Geometry check sheet. Reference: drawing and pictorial views, mm from the part's lowest x, y, z. Give positions to 0.01 mm unless a question says otherwise; leave off trailing zeros. Order: outer loops, then holes, each group sorted by start corner. A loop starts at its lowest first (then second) coordinate and runs counter-clockwise, first axis right, second up. Notation, with made-up numbers: M 63.5,76 L 83.5,76 A33 cw 83.5,111 Z; hole C -25.5,13 d9. An arc over 180 degrees is marked long. Answer as CSV lines item,"result".
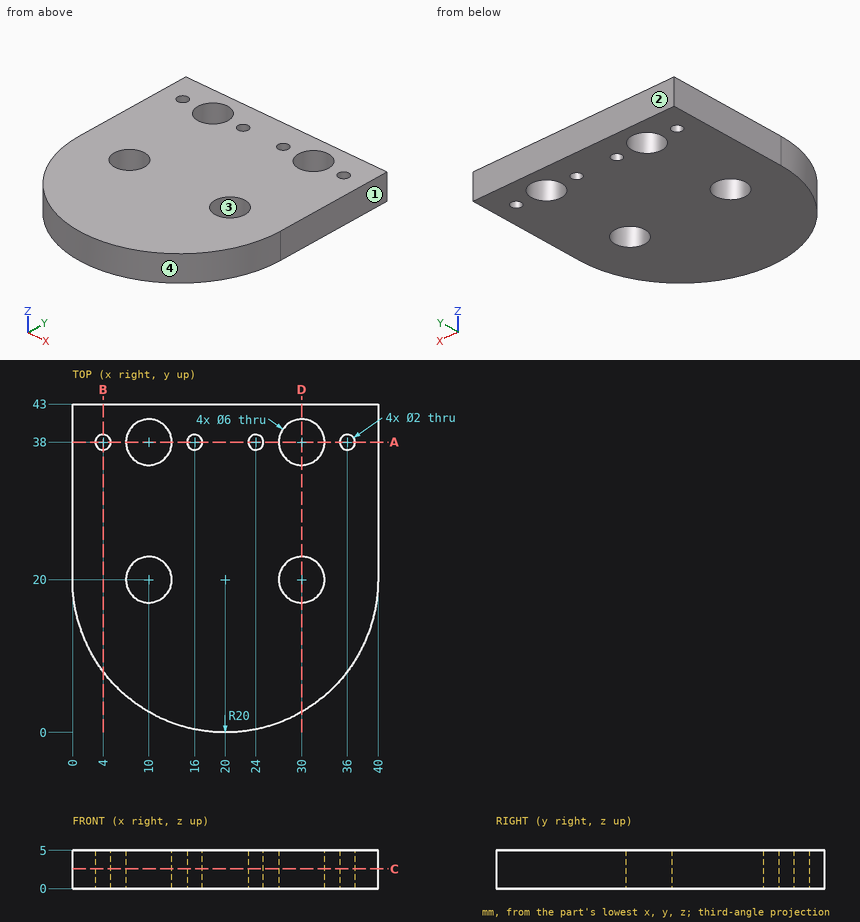
(1) Section check C-C on z = 2.6. State how many separate pieces and enclosed holes the cut face has, then the cut area to 3 significant figures.
The answers:
separate pieces,"1"
enclosed holes,"8"
area,"1,420 mm2"
(2) Section check A-A on y = 38. Enter the section's corners in (x, z).
The answers:
outline,"M 0,0 L 3,0 L 3,5 L 0,5 Z; M 5,0 L 7,0 L 7,5 L 5,5 Z; M 13,0 L 15,0 L 15,5 L 13,5 Z; M 17,0 L 23,0 L 23,5 L 17,5 Z; M 25,0 L 27,0 L 27,5 L 25,5 Z; M 33,0 L 35,0 L 35,5 L 33,5 Z; M 37,0 L 40,0 L 40,5 L 37,5 Z"
(3) Draft check along X on the marked faces 1, 2, 3 and 4. Enter one of: +X half, -X half, draft (parallel to the pull), parting line (faces both ways), or undercut.
The answers:
face 1,"+X half"
face 2,"draft"
face 3,"undercut"
face 4,"parting line"
(4) Section check B-B on x = 4. Enter the section's corners in (y, z).
The answers:
outline,"M 8,0 L 37,0 L 37,5 L 8,5 Z; M 39,0 L 43,0 L 43,5 L 39,5 Z"
(5) Section check D-D on x = 30. Enter the section's corners in (y, z), then the cut area to 3 significant figures.
The answers:
outline,"M 2.68,0 L 17,0 L 17,5 L 2.68,5 Z; M 23,0 L 35,0 L 35,5 L 23,5 Z; M 41,0 L 43,0 L 43,5 L 41,5 Z"
area,"142 mm2"
(6) Gauge pin test, flat ends, axial feed: P1, Ø1, axis at x = 33.5, z = 2.5, coming from the -Y side; P2, Ø2, axis at x = 5.5, z = 1, coming from the -Y side. Record the tip position at first contact, or that the pin passes through.
The answers:
P1,"stops at y = 4.8"
P2,"stops at y = 5.24"
(7) Material ranges on line 1 (X direction, y = 18, z = 3.35); line 2 (Y direction, x = 11, z = 3.95); line 3 (Y direction, x = 10, z = 2.5), recorded low to high.
The answers:
line 1,"x = 0.1 to 7.76, 12.24 to 27.76, 32.24 to 39.9"
line 2,"y = 2.14 to 17.17, 22.83 to 35.17, 40.83 to 43"
line 3,"y = 2.68 to 17, 23 to 35, 41 to 43"
